```python
from build123d import *

# Parameters (mm, degrees)
SKETCH1_W           = 25.4
SKETCH1_H           = 11.7
BOSS_EXTRUDE1_DEPTH = 6.35
SKETCH2_W           = 6.2
SKETCH2_H           = 9.2
CUT_EXTRUDE1_DEPTH  = 20.664581181
CUT_EXTRUDE2_DEPTH  = 20.664581181
SKETCH4_W           = 6.2
SKETCH4_H           = 9.2
CUT_EXTRUDE3_DEPTH  = 20.664581181
SKETCH5_W           = 0.25
SKETCH5_H           = 1.5
BOSS_EXTRUDE2_DEPTH = 6.5
SKETCH6_W           = 0.25
SKETCH6_H           = 1.5
BOSS_EXTRUDE3_DEPTH = 6.5
SKETCH7_W           = 0.25
SKETCH7_H           = 1.5
BOSS_EXTRUDE4_DEPTH = 6.5
SKETCH8_W           = 0.25
SKETCH8_H           = 1.5
BOSS_EXTRUDE5_DEPTH = 6.5
HOLE1_D             = 3.2
HOLE1_DEPTH         = 9
HOLE2_D             = 3.2
HOLE2_DEPTH         = 9
HOLE3_D             = 2.5
HOLE3_DEPTH         = 4.7
HOLE4_D             = 2.5
HOLE4_DEPTH         = 19.2
FILLET1_R           = 0.1
FILLET2_R           = 0.1


with BuildPart() as part:
    # Sketch1 → Boss-Extrude1 (new body)
    with BuildSketch(Plane.XZ.offset(1.08911007)):
        with Locations((1.7735363, 5.85)):
            Rectangle(SKETCH1_W, SKETCH1_H)
    extrude(amount=-BOSS_EXTRUDE1_DEPTH)

    # Sketch2 → Cut-Extrude1 (cut, through all)
    with BuildSketch(Plane(origin=(0, 5.26088993, 0), x_dir=(-1, 0, 0), z_dir=(0, 1, 0))):
        with Locations((-11.3735363, 7.1)):
            Rectangle(SKETCH2_W, SKETCH2_H)
    extrude(amount=-CUT_EXTRUDE1_DEPTH, mode=Mode.SUBTRACT)

    # Sketch3 → Cut-Extrude2 (cut, through all)
    with BuildSketch(Plane(origin=(0, 5.26088993, 0), x_dir=(-1, 0, 0), z_dir=(0, 1, 0))):
        with BuildLine():
            Line((-3.5735363, 11.7), (-3.5735363, 4.3))
            ThreePointArc((-3.5735363, 4.3), (-1.7735363, 2.5), (0.0264637, 4.3))
            Line((0.0264637, 4.3), (0.0264637, 11.7))
            Line((0.0264637, 11.7), (-3.5735363, 11.7))
        make_face()
    extrude(amount=-CUT_EXTRUDE2_DEPTH, mode=Mode.SUBTRACT)

    # Sketch4 → Cut-Extrude3 (cut, through all)
    with BuildSketch(Plane(origin=(0, 5.26088993, 0), x_dir=(-1, 0, 0), z_dir=(0, 1, 0))):
        with Locations((7.8264637, 7.1)):
            Rectangle(SKETCH4_W, SKETCH4_H)
    extrude(amount=-CUT_EXTRUDE3_DEPTH, mode=Mode.SUBTRACT)

    # Sketch5 → Boss-Extrude2 (add)
    with BuildSketch(Plane(origin=(0, 0, 0), x_dir=(-1, 0, 0), z_dir=(0, 0, -1))):
        with Locations((2.0364637, 0.81588993)):
            Rectangle(SKETCH5_W, SKETCH5_H)
    extrude(amount=BOSS_EXTRUDE2_DEPTH)

    # Sketch6 → Boss-Extrude3 (add)
    with BuildSketch(Plane(origin=(0, 0, 0), x_dir=(-1, 0, 0), z_dir=(0, 0, -1))):
        with Locations((2.0364637, 3.35588993)):
            Rectangle(SKETCH6_W, SKETCH6_H)
    extrude(amount=BOSS_EXTRUDE3_DEPTH)

    # Sketch7 → Boss-Extrude4 (add)
    with BuildSketch(Plane(origin=(0, 0, 0), x_dir=(-1, 0, 0), z_dir=(0, 0, -1))):
        with Locations((-5.5835363, 3.35588993)):
            Rectangle(SKETCH7_W, SKETCH7_H)
    extrude(amount=BOSS_EXTRUDE4_DEPTH)

    # Sketch8 → Boss-Extrude5 (add)
    with BuildSketch(Plane(origin=(0, 0, 0), x_dir=(-1, 0, 0), z_dir=(0, 0, -1))):
        with Locations((-5.5835363, 0.81588993)):
            Rectangle(SKETCH8_W, SKETCH8_H)
    extrude(amount=BOSS_EXTRUDE5_DEPTH)

    # Hole1
    with Locations(Plane.XY.offset(2.5)):
        with Locations((11.2735363, 2.08588993)):
            Hole(HOLE1_D / 2, depth=HOLE1_DEPTH)

    # Hole2
    with Locations(Plane.XY.offset(2.5)):
        with Locations((-7.7264637, 2.08588993)):
            Hole(HOLE2_D / 2, depth=HOLE2_DEPTH)

    # Hole3
    with Locations(Plane.ZY.offset(4.7264637)):
        with Locations((8.6, 2.08588993)):
            Hole(HOLE3_D / 2, depth=HOLE3_DEPTH)

    # Hole4
    with Locations(Plane(origin=(8.2735363, 0, 0), x_dir=(0, 0, -1), z_dir=(1, 0, 0))):
        with Locations((-8.6, 2.08588993)):
            Hole(HOLE4_D / 2, depth=HOLE4_DEPTH)

    # Fillet1
    fillet1_edges = [part.edges().sort_by_distance(p)[0] for p in [
        (-4.7264637, 2.08588993, 2.5),
    ]]
    fillet(fillet1_edges, radius=FILLET1_R)

    # Fillet2
    fillet2_edges = [part.edges().sort_by_distance(p)[0] for p in [
        (8.2735363, 2.08588993, 2.5),
    ]]
    fillet(fillet2_edges, radius=FILLET2_R)


solid = part.part
```
Here's how the part is built. I have some questions about the finished solid (model axes, mm). A direction names the side the tool comes from. Coordinates: 2 decimals unless noted, no trailing zeros. Write each loop counter-clockwise with the first axis right and the second up, starting at its lowest first coordinate (ties: lowest second). Pieces come first, ordered by that corner, then holes. Notation, with made-up numbers: (57.25, 22.5) - (93.25, 22.5) arc R9 cw to (93.25, 31.5) - close; hole circle Ø11 at (87, -15.75). An arc over 180 degrees is marked (long way). One line per item, written item: value.
1) I'm going to push flat-ended pins straight in: P1, Ø1.5, axis at x = 8, y = 0, coming from the -Z side; P2, Ø1.9, axis at y = 1.5, z = 9.5, coming from the -X side; P3, Ø3, axis at y = 2.09, z = 8.6, coming from the +X side. Where does each tip first touch, or does it pass through?
Model answer:
P1: stops at z = 0
P2: stops at x = -4.73
P3: stops at x = 8.27
2) Suppose I cut it at D-D on z = 1. Write out the boundary of the cut face in (x, y), and give its area (3 significant figures).
Model answer:
outline: (-10.93, -1.09) - (14.47, -1.09) - (14.47, 5.26) - (-10.93, 5.26) - close; hole circle Ø3.2 at (-7.73, 2.09); hole circle Ø3.2 at (11.27, 2.09)
area: 145 mm²
3) Suppose I cut it at C-C on x = 10.75. Write out the boundary of the cut face in (y, z).
Model answer:
outline: (-1.09, 0) - (0.57, 0) - (0.57, 2.5) - (-1.09, 2.5) - close; (3.6, 0) - (5.26, 0) - (5.26, 2.5) - (3.6, 2.5) - close
4) I need wall thicknesses on line 1 along X through (y, z) = (1.75, 10); line 2 along X through (y, z) = (0, 3.5); line 3 along Y through (x, z) = (5.75, 8.6). Which ranges of each line are inside material? Lowest first, please.
Model answer:
line 1: x = -4.73 to -0.03, 3.57 to 8.27
line 2: x = -4.73 to 0.16, 3.39 to 8.27
line 3: y = -1.09 to 0.84, 3.34 to 5.26
5) Suppose I cut it at A-A on z = 10.25. Write out the boundary of the cut face in (x, y).
Model answer:
outline: (-4.73, -1.09) - (-0.03, -1.09) - (-0.03, 5.26) - (-4.73, 5.26) - close; (3.57, -1.09) - (8.27, -1.09) - (8.27, 5.26) - (3.57, 5.26) - close
6) Suppose I cut it at B-B on y = -0.5. Write out the boundary of the cut face in (x, z), and give its area (3 significant figures).
Model answer:
outline: (-10.93, 0) - (14.47, 0) - (14.47, 2.5) - (8.37, 2.5) arc R0.1 cw to (8.27, 2.6) - (8.27, 11.7) - (3.57, 11.7) - (3.57, 4.3) arc R1.8 cw to (-0.03, 4.3) - (-0.03, 11.7) - (-4.73, 11.7) - (-4.73, 2.6) arc R0.1 cw to (-4.83, 2.5) - (-10.93, 2.5) - close
area: 151 mm²
7) We'd pull the mould along Y, two halves only. Please class faces 1 (the flat face through (-10.926, 2, 1)), 2 (the cylindrical face through (5.89, 3.14, 9.27)), 3 (the flat face through (-1, 5.261, 5)): pulls with the +Y half, pulls with the -Y half, needs draft (parallel to the pull), parting line crosses it, or undercut.
Model answer:
face 1: needs draft
face 2: undercut
face 3: pulls with the +Y half
8) On a 3-axis mill with a long thin cutter (end or side, diameter ignored), from which of +Z, -Z, +X, -X, +Y, -Y can I reach the whole of each face in a straight line? I mean faces 4 (the flat face through (8.274, 2, 7)), 5 (the flat face through (-1.911, 3, -3)), 6 (the flat face through (-4.726, 2, 7)), 7 (the flat face through (-2.161, 3, -3)), 8 (the flat face through (5.709, 3, -3)). Say none if no direction works.
Model answer:
face 4: +Z, +X, +Y, -Y
face 5: -Z, +Y, -Y
face 6: +Z, -X, +Y, -Y
face 7: -Z, -X, +Y, -Y
face 8: -Z, +X, +Y, -Y
